Can you work these out from the drawing? Everything is in mm from the part's minimum corner. A direction names the side the tool comes from. Give positions to 0.01 mm unless a question says otherwise; leave off trailing zeros. Order: outer loops, then holes, each group sorted by start corner. A loop starts at its lowest first (then second) coordinate and runs counter-clockwise, first axis right, second up. Notation, with made-up numbers: M 12.25,48 L 54.25,48 A18 ccw 54.25,75 Z; hole C 54,88 d4. An arc over 180 degrees is marked long. Answer in a Markdown table with one row per item. Add a question column.
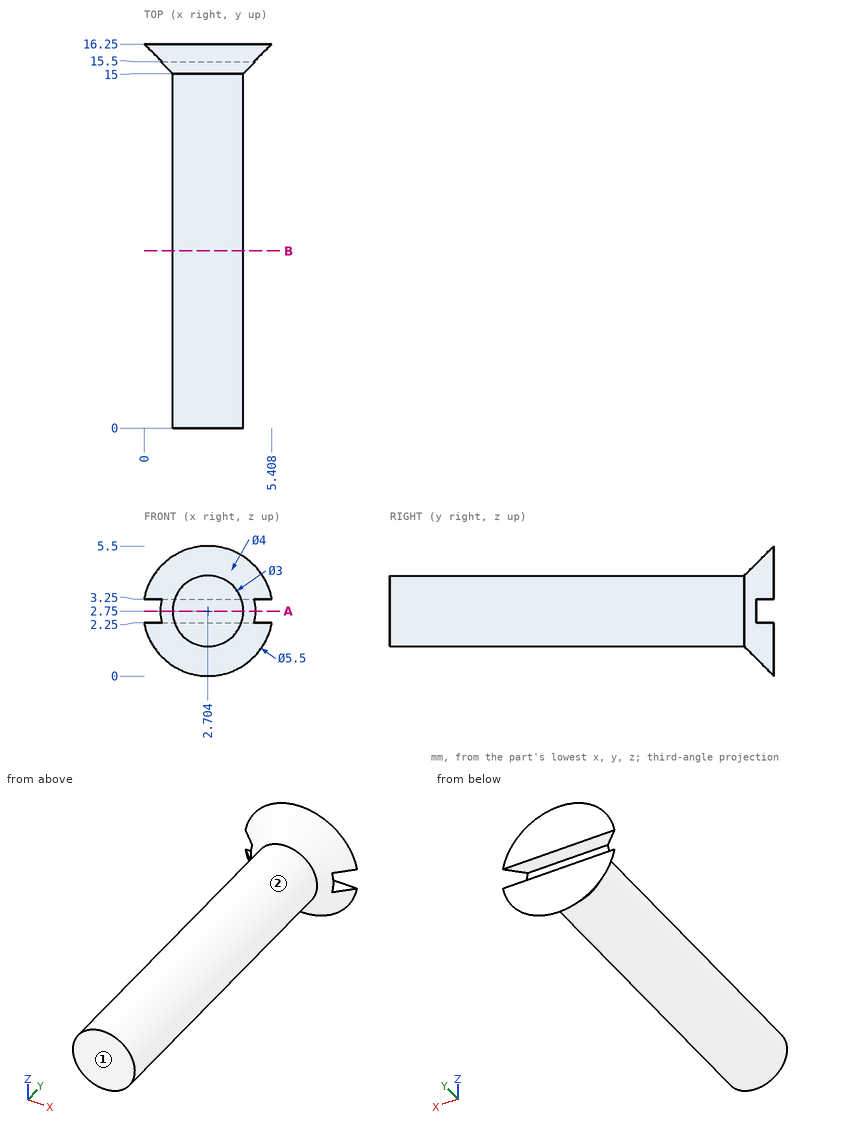
1. Suppose I cut it at A-A on z = 2.75. List the corners of the cut face in (x, y) for me.
2. For the marked faces 1 and 2, which set-ups out of +Z, -Z, +X, -X, +Y, -Y let a thin tool reach every point of the face, with its end or its side?
3. Will these pins go through, and if not, where does the flat tip stop? P1, Ø0.6, axis at x = 3.5, y = 16, coming from the -Z side; P2, Ø1, axis at x = 4, y = 4, coming from the -Z side.
4. If I drill on line 1 along Y through (x, z) = (4, 3.7); line 2 along X through (y, z) = (8.5, 3.4) (1 decimal); line 3 along Z through (x, y) = (2.9, 1.5), over which ranges is the centre line in solid material (lowest first)? Write a range as [from, to].
5. Suppose I cut it at B-B on y = 7.5. List the corners of the cut face in (x, z) for me.
Findings below:
| question | item | result |
|---|---|---|
| 1 | outline | M 0.7,15.5 L 1.2,15 L 1.2,0 L 4.2,0 L 4.2,15 L 4.7,15.5 Z |
| 2 | face 1 | +Z, -Z, +X, -X, -Y |
| 2 | face 2 | -Y |
| 3 | P1 | z = 0.07 |
| 3 | P2 | z = 1.48 |
| 4 | line 1 | [15.11, 16.25] |
| 4 | line 2 | [1.4, 4.1] |
| 4 | line 3 | [1.26, 4.24] |
| 5 | outline | C 2.7,2.75 d3 |
